```python
from build123d import *

# Parameters (mm, degrees)
ESQUISSE1_W                            = 77.5
ESQUISSE1_H                            = 90
ESQUISSE1_R                            = 1.75
EXTRUSION1_DEPTH                       = 1.5
FRAISAGE_POUR_VIS_T_TE_FRAIS_E_M2_51_D = 2.59999988
ESQUISSE5_W                            = 2
ESQUISSE5_H                            = 15.5
ENL_V_MAT_EXTRU_1_DEPTH                = 102.922764876
ENL_V_MAT_EXTRU_2_REACH                = 103.923


with BuildPart() as part:
    # Esquisse1 → Extrusion1 (new body)
    with BuildSketch(Plane(origin=(0, 0, 0), x_dir=(0, 0, -1), z_dir=(1, 0, 0))):
        with Locations((-36.25, 24)):
            Rectangle(ESQUISSE1_W, ESQUISSE1_H)
        with Locations((0, -17.5)):
            Circle(ESQUISSE1_R, mode=Mode.SUBTRACT)
        with Locations((0, 12.5)):
            Circle(ESQUISSE1_R, mode=Mode.SUBTRACT)
    extrude(amount=EXTRUSION1_DEPTH)

    # Fraisage pour vis à tête fraisée M2.51 (through all)
    with Locations(Plane(origin=(1.5, 0, 0), x_dir=(0, 0, -1), z_dir=(1, 0, 0))):
        with Locations((0, 17.5), (0, -12.5), (0, 0)):
            Hole(FRAISAGE_POUR_VIS_T_TE_FRAIS_E_M2_51_D / 2)

    # Esquisse5 → Enlèv. mat.-Extru.1 (cut, through all)
    with BuildSketch(Plane.ZY):
        with Locations((3.5, 9.25)):
            Rectangle(ESQUISSE5_W, ESQUISSE5_H)
    extrude(amount=-ENL_V_MAT_EXTRU_1_DEPTH, mode=Mode.SUBTRACT)

    # Esquisse6 → Enlèv. mat.-Extru.2 (cut, up to next)
    with BuildSketch(Plane(origin=(1.5, 0, 0), x_dir=(0, 0, -1), z_dir=(1, 0, 0)), mode=Mode.PRIVATE) as enl_v_mat_extru_2_sk1:
        Polygon((-75, 69), (-75, -1), (-70, 4), (-45, 4), (-45, 64), (-40, 69), align=None)
    enl_v_mat_extru_2_tool1 = extrude(enl_v_mat_extru_2_sk1.sketch, amount=-ENL_V_MAT_EXTRU_2_REACH, mode=Mode.PRIVATE) & part.part
    # Esquisse6 → Enlèv. mat.-Extru.2 (cut, up to next)
    with BuildSketch(Plane(origin=(1.5, 0, 0), x_dir=(0, 0, -1), z_dir=(1, 0, 0)), mode=Mode.PRIVATE) as enl_v_mat_extru_2_sk2:
        Polygon((-75, -21), (-70, -21), (-75, -16), align=None)
    enl_v_mat_extru_2_tool2 = extrude(enl_v_mat_extru_2_sk2.sketch, amount=-ENL_V_MAT_EXTRU_2_REACH, mode=Mode.PRIVATE) & part.part
    # Esquisse6 → Enlèv. mat.-Extru.2 (cut, up to next)
    with BuildSketch(Plane(origin=(1.5, 0, 0), x_dir=(0, 0, -1), z_dir=(1, 0, 0)), mode=Mode.PRIVATE) as enl_v_mat_extru_2_sk3:
        Polygon((2.5, 69), (2.5, 64), (-2.5, 69), align=None)
    enl_v_mat_extru_2_tool3 = extrude(enl_v_mat_extru_2_sk3.sketch, amount=-ENL_V_MAT_EXTRU_2_REACH, mode=Mode.PRIVATE) & part.part
    add(enl_v_mat_extru_2_tool1.solids().sort_by_distance((1.5, 36.478903, 59.978903))[0], mode=Mode.SUBTRACT)
    add(enl_v_mat_extru_2_tool2.solids().sort_by_distance((1.5, -19.333333, 73.333333))[0], mode=Mode.SUBTRACT)
    add(enl_v_mat_extru_2_tool3.solids().sort_by_distance((1.5, 67.333333, -0.833333))[0], mode=Mode.SUBTRACT)


solid = part.part
```
For this review, take the finished solid that the model builds, in its own axes (mm). Round coordinates to 2 decimals unless told otherwise and drop trailing zeros. Write each loop counter-clockwise with the first axis right and the second up, starting at its lowest first coordinate (ties: lowest second). Pieces come first, ordered by that corner, then holes.
1) Mouldability with a two-part tool opening along Y and no side actions: class faces 1 (the face through (0.74, -0.79, -1.03)), 2 (the face through (1, -19, 72)), 3 (the face through (1, 66, 43)) as +Y half, -Y half, draft (parallel to the pull), parting line (faces both ways), or undercut.
Answer below:
face 1: undercut
face 2: -Y half
face 3: +Y half
2) Take a section at A-A on y = 0. Give the boundary of the cut face in (x, z), then the cut area to 3 significant figures.
Answer below:
outline: (0, -2.5) - (1.5, -2.5) - (1.5, -1.3) - (0, -1.3) - close; (0, 1.3) - (1.5, 1.3) - (1.5, 74) - (0, 74) - close
area: 111 mm2
3) For line 1 along Y through (x, z) = (1.05, 0); line 2 along Z through (x, y) = (0.1, 39.5); line 3 along Y through (x, z) = (0.45, 52.5), list the stretches that pass through material, from the lowest coordinate up.
Answer below:
line 1: y = -21 to -19.25, -15.75 to -13.8, -11.2 to -1.3, 1.3 to 10.75, 14.25 to 16.2, 18.8 to 66.5
line 2: z = -2.5 to 45
line 3: y = -21 to 4
4) Take a section at C-C on y = 12.5. Give the boundary of the cut face in (x, z).
Answer below:
outline: (0, -2.5) - (1.5, -2.5) - (1.5, -1.75) - (0, -1.75) - close; (0, 1.75) - (1.5, 1.75) - (1.5, 2.5) - (0, 2.5) - close; (0, 4.5) - (1.5, 4.5) - (1.5, 45) - (0, 45) - close
5) Take a section at B-B on z = 0. Give the boundary of the cut face in (x, y), then the cut area to 3 significant figures.
Answer below:
outline: (0, -21) - (1.5, -21) - (1.5, -19.25) - (0, -19.25) - close; (0, -15.75) - (1.5, -15.75) - (1.5, -13.8) - (0, -13.8) - close; (0, -11.2) - (1.5, -11.2) - (1.5, -1.3) - (0, -1.3) - close; (0, 1.3) - (1.5, 1.3) - (1.5, 10.75) - (0, 10.75) - close; (0, 14.25) - (1.5, 14.25) - (1.5, 16.2) - (0, 16.2) - close; (0, 18.8) - (1.5, 18.8) - (1.5, 66.5) - (0, 66.5) - close
area: 109 mm2
6) Take a section at D-D on x = 0.6. Give the boundary of the cut face in (y, z), then the cut area to 3 significant figures.
Answer below:
outline: (-21, -2.5) - (64, -2.5) - (69, 2.5) - (69, 40) - (64, 45) - (4, 45) - (4, 70) - (-1, 75) - (-16, 75) - (-21, 70) - close; hole circle Ø3.5 at (-17.5, 0); hole circle Ø2.6 at (-12.5, 0); hole circle Ø2.6 at (0, 0); hole (1.5, 2.5) - (17, 2.5) - (17, 4.5) - (1.5, 4.5) - close; hole circle Ø3.5 at (12.5, 0); hole circle Ø2.6 at (17.5, 0)
area: 4,910 mm2
